The model under review builds one solid part; all positions refer to its coordinate system, in mm. A direction names the side the tool comes from. Coordinates: 2 decimals unless noted, no trailing zeros. Loops run counter-clockwise (first coordinate to the right, second up) from the corner with the lowest first, then second, coordinate; pieces in that order, holes last. Notation, with made-up numbers: (-6.75, -34.75) - (21.25, -34.75) arc R14 ccw to (21.25, -8.75) - close; hole circle Ø3 at (-3.75, 57). An arc over 180 degrees is marked (long way). One line per item, written item: value. Start each with the question number.
1. We need section D-D, the plane z = 7. Give the boundary of the cut face in (x, y).
2. We need section B-B, the plane x = -129. Give the boundary of the cut face in (y, z).
3. Mouldability with a two-part tool opening along X and no side actions: class faces 1 (the face through (-135.19, 4.93, 49.27)), 2 (the face through (-106, 7, 11)), 3 (the face through (-124, 5, 11)), 4 (the face through (-134.92, 5.07, 14.58)) as +X half, -X half, draft (parallel to the pull), parting line (faces both ways), or undercut.
4. We need section C-C, the plane y = 7. Give the boundary of the cut face in (x, z), then the cut area to 3 significant figures.
5. Insertion check: P1, Ø5, axis at x = -136, z = 18.5, coming from the +Y side; P2, Ø3.5, axis at x = -124, y = 5.5, coming from the +Z side; P3, Ø5, axis at y = 6, z = 31.5, coming from the -X side. Each pin has a flat end and moves straight along its axis. Give the tip position at first contact, or say it passes through.
6. For faces 5 (the face through (-141.618, 5, 27)), 6 (the face through (-116.025, 4.355, 11.889)), 7 (the face through (-121, 0, 26)), 8 (the face through (-133.507, 5, 41)), list the 3-axis set-ups (+Z, -Z, +X, -X, +Y, -Y) from which the entire face can be reached by the end or side of a thin tool; tool diameter is ignored.
7. To check wall thickness, follow line 1 (X direction, y = 4.75, z = 7); line 2 (X direction, y = 10.75, z = 6); line 3 (Y direction, x = -135.5, z = 47.5). State the ranges of each line that lie inside material, in increasing order.
8. We need section A-A, the plane z = 27. Give the boundary of the cut face in (x, y).
from build123d import *

# Parameters (mm, degrees)
SKETCH1_R           = 2.1
SKETCH1_R_2         = 3.05
BOSS_EXTRUDE1_DEPTH = 11
FILLET1_R           = 2.5
SKETCH2_W           = 62.859905726
SKETCH2_H           = 67.127049317
CUT_EXTRUDE1_DEPTH  = 1


with BuildPart() as part:
    # Sketch1 → Boss-Extrude1 (new body)
    with BuildSketch(Plane(origin=(0, 0, 0), x_dir=(1, 0, 0), z_dir=(0, 1, 0))):
        with BuildLine():
            Line((-141.618033146, -48.413320241), (-141.618033146, -47.605254623))
            ThreePointArc((-141.618033146, -47.605254623), (-142.400057305, -45.070169685), (-141.618033146, -42.535084747))
            Line((-141.618033146, -42.535084747), (-141.618033146, -12.337550143))
            ThreePointArc((-141.618033146, -12.337550143), (-137.391034255, -7.146662711), (-132.135747469, -3.000002276))
            Line((-132.135747469, -3.000002276), (-103.999998533, -3.000002276))
            ThreePointArc((-103.999998533, -3.000002276), (-99.999998533, -7.000002276), (-103.999998533, -11.000002276))
            Line((-103.999998533, -11.000002276), (-108.800450096, -11.000002276))
            ThreePointArc((-108.800450096, -11.000002276), (-115.958524417, -28.957739522), (-133.507162881, -37.067218112))
            Line((-133.507162881, -37.067218112), (-133.507162881, -42.428250309))
            ThreePointArc((-133.507162881, -42.428250309), (-133.376053416, -42.838619725), (-133.243682576, -43.248584005))
            ThreePointArc((-133.243682576, -43.248584005), (-135.275410049, -49.325898387), (-141.618033146, -48.413320241))
        make_face()
        with Locations(Location((-103.999998533, -7.000002276, 0), (0, 0, 270))):
            Circle(SKETCH1_R, mode=Mode.SUBTRACT)
        with Locations(Location((-120, -7, 0), (0, 0, 270))):
            Circle(SKETCH1_R, mode=Mode.SUBTRACT)
        with Locations(Location((-137.900057305, -45.070169685, 0), (0, 0, 270))):
            Circle(SKETCH1_R_2, mode=Mode.SUBTRACT)
        with BuildLine():
            Line((-115.253720534, -10.999999988), (-131.784308175, -10.999999988))
            ThreePointArc((-131.784308175, -10.999999988), (-133.51136611, -12.688858333), (-135.059388528, -14.543204098))
            Line((-135.059388528, -14.543204098), (-135.076749083, -30.65065719))
            ThreePointArc((-135.076749083, -30.65065719), (-121.070294848, -24.956188484), (-115.253720534, -10.999999988))
        make_face(mode=Mode.SUBTRACT)
    extrude(amount=BOSS_EXTRUDE1_DEPTH)

    # Fillet1
    fillet1_edges = [part.edges().sort_by_distance(p)[0] for p in [
        (-141.618033146, 5.5, 42.535084747),
        (-132.135747469, 5.5, 3.000002276),
        (-108.800450096, 5.5, 11.000002276),
        (-133.507162881, 5.5, 37.067218112),
        (-133.507162881, 5.5, 42.428250309),
        (-133.243682576, 5.5, 43.248584005),
        (-141.618033146, 5.5, 47.605254623),
        (-135.076749083, 5.5, 30.65065719),
        (-115.253720534, 5.5, 10.999999988),
        (-131.784308175, 5.5, 10.999999988),
        (-135.059388528, 5.5, 14.543204098),
    ]]
    fillet(fillet1_edges, radius=FILLET1_R)

    # Sketch2 → Cut-Extrude1 (cut)
    with BuildSketch(Plane(origin=(0, 11, 0), x_dir=(1, 0, 0), z_dir=(0, 1, 0))):
        with Locations((-133.229918527, -44.563526935)):
            Rectangle(SKETCH2_W, SKETCH2_H)
    extrude(amount=-CUT_EXTRUDE1_DEPTH, mode=Mode.SUBTRACT)


solid = part.part
Findings below:
1. outline: (-137.24, 0) - (-122.1, 0) - (-122.1, 11) - (-137.24, 11) - close; (-117.9, 0) - (-106.1, 0) - (-106.1, 11) - (-117.9, 11) - close; (-101.9, 0) - (-100, 0) - (-100, 11) - (-101.9, 11) - close
2. outline: (0, 3) - (11, 3) - (11, 11) - (0, 11) - close; (0, 29.74) - (10, 29.74) - (10, 36.43) - (0, 36.43) - close
3. face 1: parting line
3. face 2: draft
3. face 3: undercut
3. face 4: undercut
4. outline: (-141.9, 43) arc R2.5 cw to (-141.62, 41.86) - (-141.62, 12.34) arc R30.58 ccw to (-132.78, 3.41) arc R2.5 ccw to (-131.4, 3) - (-104, 3) arc R4 ccw to (-104, 11) - (-106.41, 11) arc R2.5 cw to (-108.9, 13.28) arc R26.1 ccw to (-131.35, 36.86) arc R2.5 cw to (-133.51, 39.34) - (-133.51, 42.04) arc R2.5 cw to (-133.39, 42.8) arc R140.09 cw to (-133.24, 43.25) arc R5 ccw to (-141.62, 48.41) - (-141.62, 48.29) arc R2.5 cw to (-141.9, 47.14) arc R4.5 ccw to start; hole circle Ø6.1 at (-137.9, 45.07); hole (-135.07, 27.99) - (-135.06, 15.4) arc R2.5 ccw to (-134.5, 13.83) arc R23.93 ccw to (-132.54, 11.7) arc R2.5 ccw to (-130.81, 11) - (-117.94, 11) arc R2.5 ccw to (-115.46, 13.86) arc R19.65 ccw to (-132.23, 30.47) arc R2.5 ccw to start; hole circle Ø4.2 at (-120, 7); hole circle Ø4.2 at (-104, 7)
4. area: 751 mm2
5. P1: y = 10
5. P2: z = 35.45
5. P3: x = -141.62
6. face 5: -Z, -X, +Y, -Y
6. face 6: +Y, -Y
6. face 7: +Z, -Z, +X, -X, -Y
6. face 8: +X, +Y, -Y
7. line 1: -137.24 to -122.1, -117.9 to -106.1, -101.9 to -100
7. line 2: -136.16 to -121.85, -118.15 to -105.85, -102.15 to -100.13
7. line 3: 0 to 10
8. outline: (-141.62, 0) - (-135.07, 0) - (-135.07, 10) - (-141.62, 10) - close; (-123.5, 0) - (-114.28, 0) - (-114.28, 10) - (-123.5, 10) - close
